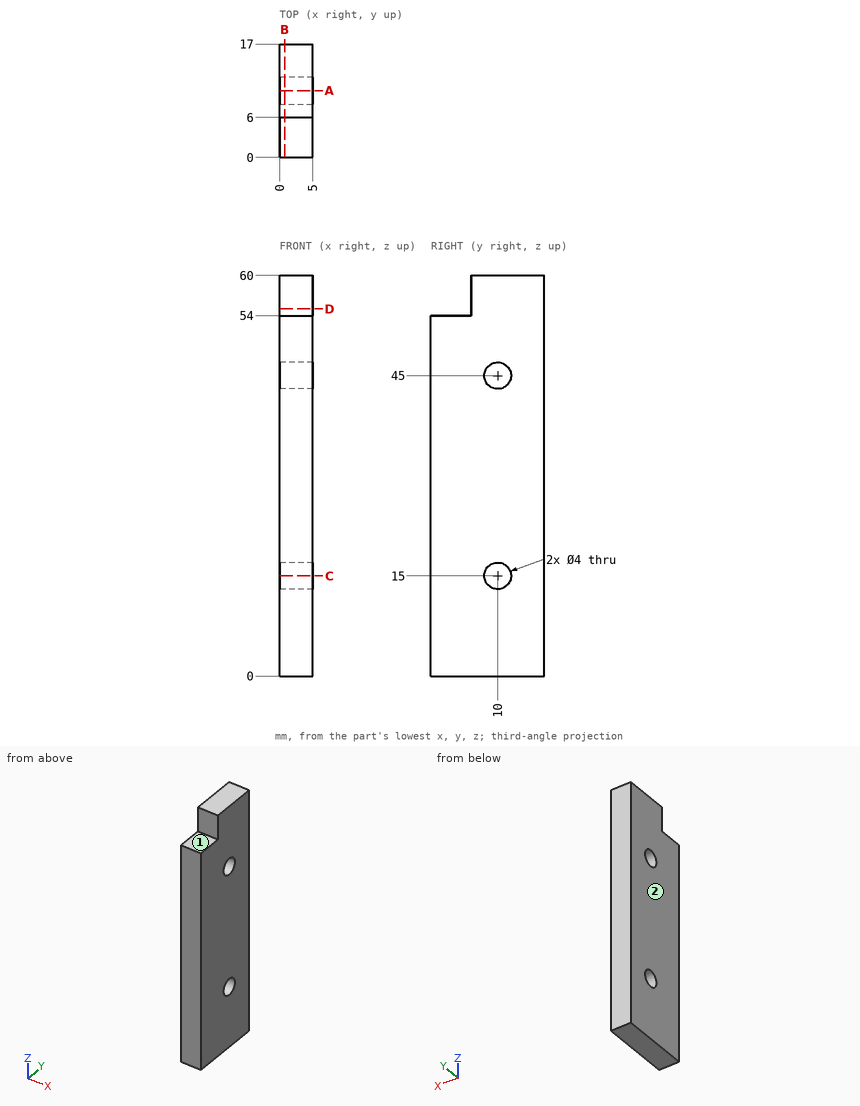
For this review, use the dimensioned drawing (mm, ordinates from the lowest corner) and the shaded views. A direction names the side the tool comes from. Coordinates: 2 decimals unless noted, no trailing zeros. Loops run counter-clockwise (first coordinate to the right, second up) from the corner with the lowest first, then second, coordinate; pieces in that order, holes last. Notation, with made-up numbers: (58.5, 81.25) - (75.5, 81.25) arc R22 ccw to (75.5, 114.25) - close; hole circle Ø7 at (-2.5, 33). An arc over 180 degrees is marked (long way). Use CSV: the item, a comma, the result in double quotes. Start each with the question number.
1) Consider section C-C on z = 15. Write out the cut boundary in (x, y).
2) Consider section B-B on x = 0.75. Write out the cut boundary in (y, z).
3) Consider section D-D on z = 55. Write out the cut boundary in (x, y), then the cut area to 3 significant figures.
4) For pin 1 Ø1.5 at (x, z) = (1.5, 57.5) entering from -Y, flat-tipped, find the tip position at first contact; note if it passes through.
5) Wall thickness on L1, parallel to Z at x = 3.25, y = 10; L2, parallel to Z at x = 1, y = 4.25; L3, parallel to Z at x = 1.1, y = 9.5: over which ranges is each line inside the solid? List them lowest first. Write a range as from..to.
6) Tool access review of the marked faces 1 and 2: name each direction out of +Z, -Z, +X, -X, +Y, -Y from which nothing blocks a thin tool from reaching the whole face with its end or side.
7) Consider section A-A on y = 10. Write out the cut boundary in (x, z), then the cut area to 3 significant figures.
Geometry says:
1,outline,"(0, 0) - (5, 0) - (5, 8) - (0, 8) - close; (0, 12) - (5, 12) - (5, 17) - (0, 17) - close"
2,outline,"(0, 0) - (17, 0) - (17, 60) - (6, 60) - (6, 54) - (0, 54) - close; hole circle Ø4 at (10, 15); hole circle Ø4 at (10, 45)"
3,outline,"(0, 6) - (5, 6) - (5, 17) - (0, 17) - close"
3,area,"55.0 mm^2"
4,pin 1,"y = 6"
5,L1,"0..13, 17..43, 47..60"
5,L2,"0..54"
5,L3,"0..13.06, 16.94..43.06, 46.94..60"
6,face 1,"+Z, +X, -X, -Y"
6,face 2,"+Z, -Z, -X, +Y, -Y"
7,outline,"(0, 0) - (5, 0) - (5, 13) - (0, 13) - close; (0, 17) - (5, 17) - (5, 43) - (0, 43) - close; (0, 47) - (5, 47) - (5, 60) - (0, 60) - close"
7,area,"260 mm^2"
